Check sheet for the modelled part. Datum: model origin and axes. Units: mm. Face numbers are marked on the shaded views. Coordinates: 2 decimals unless noted, no trailing zeros. Loops run counter-clockwise (first coordinate to the right, second up) from the corner with the lowest first, then second, coordinate; pieces in that order, holes last. Notation, with made-up numbers: (75.25, -8) -> (115.25, -8) arc R23 ccw to (115.25, 15) -> close; hole circle Ø10 at (-22, -28). An arc over 180 degrees is marked (long way). Use CSV: the item, a comma, the result in double quotes. Start each with the question number.
1. Sectioned sample at C-C, the plane y = -221.5. Record the cut outline in (x, z), and give its area (3 significant figures).
2. Thickness scan on L1, parallel to Z at x = -13.5, y = -221.5; L2, parallel to X at y = 183, z = 5; L3, parallel to Y at x = 29, z = -14.4. Record the ranges inside material, lowest first.
3. Gauge pin test, flat ends, axial feed: pin 1 (12.5 mm diameter, centred on y = -234.5, z = 3.5, fed in from +X); pin 2 (10 mm diameter, centred on x = 44.5, y = -20.5, fed in from +Z); pin 3 (12.5 mm diameter, centred on y = 44, z = -5.5, fed in from -X); pin 4 (12 mm diameter, centred on y = -125, z = -8.5, fed in from +X). Record the tip position at first contact, or that the pin passes through.
4. Release check for a two-part mould opening along Z. For the marked faces 1, 2 and 3 record: pulls with the +Z half, pulls with the -Z half, needs draft (parallel to the pull), parting line crosses it, or undercut.
5. Sectioned sample at A-A, the plane z = -6.5. Count the separate pieces of the cut face and the enclosed holes in it, and give its area (3 significant figures).
6. Sectioned sample at B-B, the plane y = 130. Record the cut outline in (x, z).
7. Sectioned sample at D-D, the plane x = -38.5. Record the cut outline in (y, z), and give its area (3 significant figures).
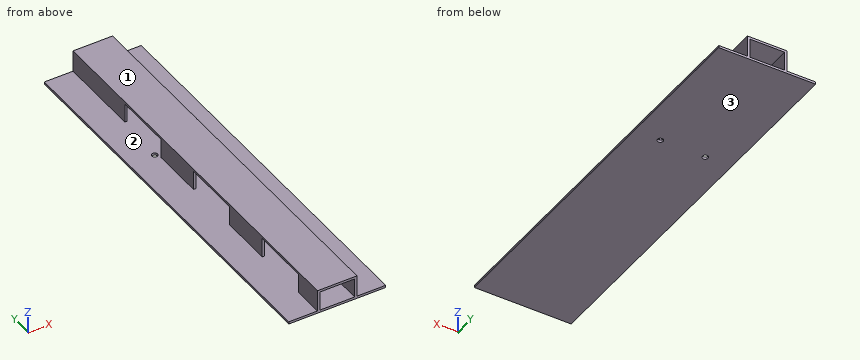
```python
from build123d import *

# Parameters (mm, degrees)
CROQUIS1_W                 = 51
CROQUIS1_H                 = 31
CROQUIS1_W_2               = 45
CROQUIS1_H_2               = 25
SALIENTE_EXTRUIR2_DEPTH    = 254.5
CROQUIS3_W                 = 25
CROQUIS3_H                 = 75
CORTAR_EXTRUIR1_DEPTH      = 1
CORTAR_EXTRUIR1_DEPTH_BACK = 52
CROQUIS4_W                 = 37
CROQUIS4_H                 = 509
SALIENTE_EXTRUIR3_DEPTH    = 3
CORTAR_EXTRUIR2_START      = -4
CROQUIS5_R                 = 3.75
CORTAR_EXTRUIR2_DEPTH      = 33


with BuildPart() as part:
    # Croquis1 → Saliente-Extruir2 (new body, symmetric)
    with BuildSketch(Plane(origin=(0, 0, 0), x_dir=(1, 0, 0), z_dir=(0, 1, 0))):
        Rectangle(CROQUIS1_W, CROQUIS1_H)
        Rectangle(CROQUIS1_W_2, CROQUIS1_H_2, mode=Mode.SUBTRACT)
    extrude(amount=SALIENTE_EXTRUIR2_DEPTH, both=True)

    # Croquis3 → Cortar-Extruir1 (cut, two sides)
    with BuildSketch(Plane(origin=(25.5, 0, 0), x_dir=(0, 0, -1), z_dir=(1, 0, 0))) as cortar_extruir1_sk:
        with Locations((0, 109)):
            Rectangle(CROQUIS3_W, CROQUIS3_H)
        with Locations((0, -34)):
            Rectangle(CROQUIS3_W, CROQUIS3_H)
        with Locations((0, -177)):
            Rectangle(CROQUIS3_W, CROQUIS3_H)
    extrude(amount=CORTAR_EXTRUIR1_DEPTH, mode=Mode.SUBTRACT)
    extrude(cortar_extruir1_sk.sketch, amount=-CORTAR_EXTRUIR1_DEPTH_BACK, mode=Mode.SUBTRACT)

    # Croquis4 → Saliente-Extruir3 (add)
    with BuildSketch(Plane(origin=(0, 0, -15.5), x_dir=(-1, 0, 0), z_dir=(0, 0, -1))):
        with Locations((-44, 0)):
            Rectangle(CROQUIS4_W, CROQUIS4_H)
        with Locations((44, 0)):
            Rectangle(CROQUIS4_W, CROQUIS4_H)
    extrude(amount=-SALIENTE_EXTRUIR3_DEPTH)

    # Croquis5 → Cortar-Extruir2 (cut)
    with BuildSketch(Plane.XY.offset(-12.5).offset(CORTAR_EXTRUIR2_START)):
        with Locations((-29, 78.693747285)):
            Circle(CROQUIS5_R)
    cortar_extruir2 = extrude(amount=CORTAR_EXTRUIR2_DEPTH, mode=Mode.SUBTRACT)

    # Simetría1: Cortar-Extruir2 across plane
    add(cortar_extruir2.mirror(Plane(origin=(0, 0, 0), x_dir=(0, 0, 1), z_dir=(1, 0, 0))), mode=Mode.SUBTRACT)


solid = part.part
```
Completed:
1,outline,"(-62.5, -15.5) -> (62.5, -15.5) -> (62.5, -12.5) -> (25.5, -12.5) -> (25.5, 15.5) -> (-25.5, 15.5) -> (-25.5, -12.5) -> (-62.5, -12.5) -> close; hole (-22.5, -12.5) -> (22.5, -12.5) -> (22.5, 12.5) -> (-22.5, 12.5) -> close"
1,area,"678 mm²"
2,L1,"-15.5 to -12.5, 12.5 to 15.5"
2,L2,"-25.5 to -22.5, 22.5 to 25.5"
2,L3,"-254.5 to 74.94, 82.44 to 254.5"
3,pin 1,"x = 25.5"
3,pin 2,"z = -12.5"
3,pin 3,"x = -25.5"
3,pin 4,"x = 62.5"
4,face 1,"pulls with the +Z half"
4,face 2,"undercut"
4,face 3,"pulls with the -Z half"
5,separate pieces,"8"
5,enclosed holes,"0"
5,area,"1,700 mm²"
6,outline,"(-62.5, -15.5) -> (62.5, -15.5) -> (62.5, -12.5) -> (-62.5, -12.5) -> close; (-25.5, 12.5) -> (25.5, 12.5) -> (25.5, 15.5) -> (-25.5, 15.5) -> close"
7,outline,"(-254.5, -15.5) -> (254.5, -15.5) -> (254.5, -12.5) -> (-254.5, -12.5) -> close"
7,area,"1,530 mm²"
